The model under review builds one solid part; all positions refer to its coordinate system, in mm. A direction names the side the tool comes from. Coordinates: 2 decimals unless noted, no trailing zeros. Write each loop counter-clockwise with the first axis right and the second up, starting at its lowest first coordinate (ties: lowest second). Pieces come first, ordered by that corner, then holes. Notation, with made-up numbers: (63, 68) - (68, 68) arc R19 ccw to (68, 101) - close; hole circle Ø10 at (-9.5, -37.75). An arc over 180 degrees is marked (long way). Put each result on its own line as item: value. Start each with the question number.
Item 1: Consider section B-B on y = 0. Give the boundary of the cut face in (x, z), then the cut area to 3 significant figures.
Item 2: Machinability: for faces 4 (the face through (5.035, 48.515, 14.79)), 5 (the face through (-4.97, 48.42, 14.79)), 6 (the face through (40.2, 13.5, 30)), which of the approach directions +Z, -Z, +X, -X, +Y, -Y give a long, thin tool a straight path to every point of the face, cutting with its end or side? Answer none if there is none.
Item 3: To check wall thickness, follow L1, parallel to Y at x = 0, z = 19; L2, parallel to Y at x = 3.5, z = 21; L3, parallel to X at y = 14.5, z = 3.5. State the ranges of each line that lie inside material, in increasing order. Write a range as [from, to].
Item 4: For pin 1 (2 mm diameter, centred on x = -15.5, z = 18.5, fed in from -Y); pin 2 (5 mm diameter, centred on x = -31.5, y = 25.5, fed in from +Z); pin 3 (2 mm diameter, centred on x = -11, z = 13.5, fed in from +Y); pin 4 (10 mm diameter, centred on x = -7, z = 11.5, fed in from -Y), all flat-tipped, find the tip position at first contact; note any pin that passes through.
Item 5: Consider section C-C on z = 3. Give the boundary of the cut face in (x, y), then the cut area to 3 significant figures.
Item 6: Consider section A-A on x = 0. Give the boundary of the cut face in (y, z), then the cut area to 3 significant figures.
Item 7: Consider section D-D on x = 20. Give the boundary of the cut face in (y, z), then the cut area to 3 significant figures.
Item 8: Mouldability with a two-part tool opening along Y and no side actions: class faces 1 (the face through (26.9, 32.5, 0)), 2 (the face through (40.06, 12.62, 14.79)), 3 (the face through (-0.11, 49.2, 25.73)) as pulls with the +Y half, pulls with the -Y half, needs draft (parallel to the pull), parting line crosses it, or undercut.
```python
from build123d import *

# Parameters (mm, degrees)
SKETCH1_R                      = 42
BOSS_EXTRUDE1_DEPTH            = 30
CUT_EXTRUDE1_REACH             = 47
CUT_EXTRUDE1_DIRECTION_2_REACH = 47


with BuildPart() as part:
    # Sketch1 → Boss-Extrude1 (new body)
    with BuildSketch(Plane.XY):
        with BuildLine():
            ThreePointArc((2.5, 44.930501889), (15.285447634, 42.324403016), (26.785714286, 36.159722209))
            ThreePointArc((26.785714286, 36.159722209), (-12.910485027, -43.108228639), (-2.5, 44.930501889))
            Line((-2.5, 44.930501889), (-7.5, 52))
            Line((-7.5, 52), (7.5, 52))
            Line((7.5, 52), (2.5, 44.930501889))
        make_face()
        Circle(SKETCH1_R, mode=Mode.SUBTRACT)
    extrude(amount=BOSS_EXTRUDE1_DEPTH)

    # Cut-Extrude1: up to this face of the body (flat: up to its plane)
    cut_extrude1_end = Plane(part.part.faces().sort_by_distance((-5, 48.465250945, 15))[0])
    # Sketch3 → Cut-Extrude1 (cut, up to the picked face)
    with BuildSketch(Plane(origin=(0, 0, 0), x_dir=(0, 0, -1), z_dir=(1, 0, 0)), mode=Mode.PRIVATE) as cut_extrude1_sk1:
        Polygon((-30, 44.930501889), (-22.930501889, 52), (-30, 52), align=None)
    cut_extrude1_tool1 = split(extrude(cut_extrude1_sk1.sketch, amount=-CUT_EXTRUDE1_REACH, mode=Mode.PRIVATE), bisect_by=cut_extrude1_end, keep=Keep.BOTH, mode=Mode.PRIVATE)
    add(cut_extrude1_tool1.solids().sort_by_distance((0, 49.643501, 27.643501))[0], mode=Mode.SUBTRACT)

    # Cut-Extrude1 direction 2: up to this face of the body (flat: up to its plane)
    cut_extrude1_direction_2_end = Plane(part.part.faces().sort_by_distance((5, 48.465250945, 15))[0])
    # Sketch3 → Cut-Extrude1 direction 2 (cut, up to the picked face)
    with BuildSketch(Plane(origin=(0, 0, 0), x_dir=(0, 0, -1), z_dir=(1, 0, 0)), mode=Mode.PRIVATE) as cut_extrude1_direction_2_sk1:
        Polygon((-30, 44.930501889), (-22.930501889, 52), (-30, 52), align=None)
    cut_extrude1_direction_2_tool1 = split(extrude(cut_extrude1_direction_2_sk1.sketch, amount=CUT_EXTRUDE1_DIRECTION_2_REACH, mode=Mode.PRIVATE), bisect_by=cut_extrude1_direction_2_end, keep=Keep.BOTH, mode=Mode.PRIVATE)
    add(cut_extrude1_direction_2_tool1.solids().sort_by_distance((0, 49.643501, 27.643501))[0], mode=Mode.SUBTRACT)


solid = part.part
```
Report:
1. outline: (-45, 0) - (-42, 0) - (-42, 30) - (-45, 30) - close; (42, 0) - (45, 0) - (45, 30) - (42, 30) - close
1. area: 180 mm²
2. face 4: +Z, -Z, +X
2. face 5: +Z, -Z, -X
2. face 6: +Z, +X, -X, +Y, -Y
3. L1: [-45, -42], [42, 52]
3. L2: [-44.86, -41.85], [41.85, 44.86], [46.34, 52]
3. L3: [-42.6, -39.42], [39.42, 42.6]
4. pin 1: y = -42.6
4. pin 2: z = 30
4. pin 3: y = 43.87
4. pin 4: y = -44.96
5. outline: (-7.5, 52) - (-2.5, 44.93) arc R45 ccw (long way) to (2.5, 44.93) - (7.5, 52) - close; hole circle Ø84 at (0, 0)
5. area: 890 mm²
6. outline: (-45, 0) - (-42, 0) - (-42, 30) - (-45, 30) - close; (42, 0) - (52, 0) - (52, 22.93) - (44.93, 30) - (42, 30) - close
6. area: 365 mm²
7. outline: (-40.31, 0) - (-36.93, 0) - (-36.93, 30) - (-40.31, 30) - close; (36.93, 0) - (40.31, 0) - (40.31, 30) - (36.93, 30) - close
7. area: 203 mm²
8. face 1: needs draft
8. face 2: undercut
8. face 3: pulls with the +Y half
